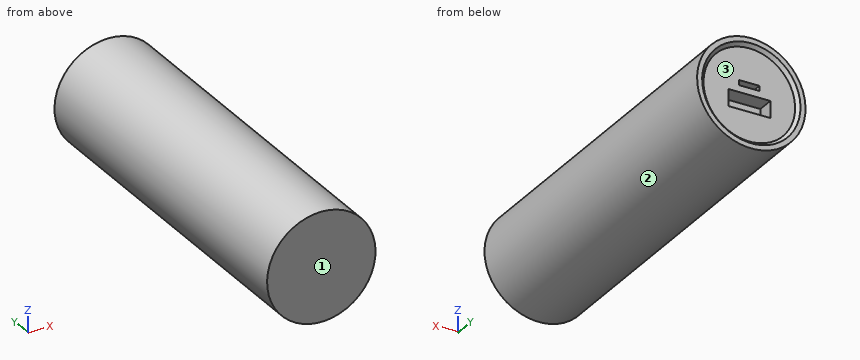
from build123d import *

# Parameters (mm, degrees)
SKETCH1_R           = 16.125
BOSS_EXTRUDE1_DEPTH = 106.9
SKETCH2_R           = 14.625
CUT_EXTRUDE1_DEPTH  = 1
CHAMFER1_SIZE       = 1
SKETCH3_W           = 12.5
SKETCH3_H           = 5
SKETCH3_W_2         = 6
SKETCH3_H_2         = 1.5
CUT_EXTRUDE2_DEPTH  = 5


with BuildPart() as part:
    # Sketch1 → Boss-Extrude1 (new body)
    with BuildSketch(Plane(origin=(0, 0, 0), x_dir=(1, 0, 0), z_dir=(0, 1, 0))):
        with Locations(Location((0, 0, 0), (0, 0, 270))):
            Circle(SKETCH1_R)
    extrude(amount=BOSS_EXTRUDE1_DEPTH)

    # Sketch2 → Cut-Extrude1 (cut)
    with BuildSketch(Plane(origin=(0, 106.9, 0), x_dir=(1, 0, 0), z_dir=(0, 1, 0))):
        with Locations(Location((0, 0, 0), (0, 0, 270))):
            Circle(SKETCH2_R)
    extrude(amount=-CUT_EXTRUDE1_DEPTH, mode=Mode.SUBTRACT)

    # Chamfer1
    chamfer1_edges = [part.edges().sort_by_distance(p)[0] for p in [
        (0, 105.9, -14.625),
    ]]
    chamfer(chamfer1_edges, length=CHAMFER1_SIZE - 0.0001)  # a hair under: the kernel refuses the full size

    # Sketch3 → Cut-Extrude2 (cut)
    with BuildSketch(Plane(origin=(0, 105.9, 0), x_dir=(1, 0, 0), z_dir=(0, 1, 0))):
        with Locations((0, 2.5)):
            Rectangle(SKETCH3_W, SKETCH3_H)
        with Locations((0, -2.75)):
            Rectangle(SKETCH3_W_2, SKETCH3_H_2)
    extrude(amount=-CUT_EXTRUDE2_DEPTH, mode=Mode.SUBTRACT)


solid = part.part
Work out the finished part from the listing and answer in its coordinate system (mm). Face numbers are marked on the shaded views. Round coordinates to 2 decimals unless told otherwise and drop trailing zeros. Loops run counter-clockwise (first coordinate to the right, second up) from the corner with the lowest first, then second, coordinate; pieces in that order, holes last. Notation, with made-up numbers: (66, 82.5) -> (79, 82.5) arc R30 ccw to (79, 121.5) -> close; hole circle Ø4 at (45, 49). An arc over 180 degrees is marked (long way). Use one line per item in the form item = value.
(1) Straight lines are drawn through the part: line 1 (Y direction, x = -4, z = 2); line 2 (X direction, y = 106, z = 0) (3 decimals); line 3 (Y direction, x = -5, z = -1). For each, find the intervals that lie inside material, in ascending order.
Answer list:
line_1 = 0 to 105.9
line_2 = -16.125 to -13.725, 13.725 to 16.125
line_3 = 0 to 100.9
(2) Flat-ended cylindrical pins translate along their axes: P1, Ø1.6, axis at y = 102, z = 2.5, coming from the +X side; P2, Ø1.5, axis at x = 5.5, y = 62.5, coming from the -Z side; P3, Ø1, axis at y = 45, z = 7.5, coming from the +X side. Find the tip coordinate at first contact, or state that the pin passes through.
Answer list:
P1 = 16.04
P2 = -15.41
P3 = 14.53
(3) Find section B-B on y = 16. Give the vertices of the cut face in (x, z) (3 decimals), then the cut area to 3 significant figures.
Answer list:
outline = circle Ø32.25 at (0, 0)
area = 817 mm2
(4) For a pull along X with two mould halves and no side action, classify the marked faces 1, 2 and 3 as released by +X, released by -X, zero draft, split by the parting line, or undercut.
Answer list:
face_1 = zero draft
face_2 = split by the parting line
face_3 = undercut
